Source: CAD feature listing. Evaluate the final solid. Frame: model axes, mm. Face numbers are marked on the shaded views. A direction names the side the tool comes from. Round coordinates to 2 decimals unless told otherwise and drop trailing zeros. Write each loop counter-clockwise with the first axis right and the second up, starting at its lowest first coordinate (ties: lowest second). Pieces come first, ordered by that corner, then holes. Notation, with made-up numbers: (1, 52) -> (11, 52) arc R16 cw to (11, 67) -> close; hole circle Ø7 at (31, 27.25). An arc over 180 degrees is marked (long way). Put each result on its own line as item: value.
```python
from build123d import *

# Parameters (mm, degrees)
BOSS_EXTRUDE1_DEPTH      = 3
BOSS_EXTRUDE2_START      = 22.115178
SKETCH3_W                = 10.4
SKETCH3_H                = 10.35
BOSS_EXTRUDE2_DEPTH      = 1
BOSS_EXTRUDE2_DEPTH_BACK = 3
CUT_EXTRUDE1_DEPTH       = 4
BOSS_EXTRUDE3_DEPTH      = 2
SKETCH6_W                = 4
SKETCH6_H                = 3.75
BOSS_EXTRUDE4_DEPTH      = 1
SKETCH7_W                = 4
SKETCH7_H                = 3.75
BOSS_EXTRUDE5_DEPTH      = 1
SKETCH8_W                = 3.8
SKETCH8_H                = 4
BOSS_EXTRUDE6_DEPTH      = 1
SKETCH9_W                = 3.8
SKETCH9_H                = 4
BOSS_EXTRUDE7_DEPTH      = 1
CUT_EXTRUDE2_DEPTH       = 3
BOSS_EXTRUDE8_DEPTH      = 3
BOSS_EXTRUDE9_DEPTH      = 6
BOSS_EXTRUDE10_DEPTH     = 7
SKETCH15_W               = 12.4
SKETCH15_H               = 12.35
CUT_EXTRUDE3_DEPTH       = 1.5


with BuildPart() as part:
    # Sketch1 → Boss-Extrude1 (new body)
    with BuildSketch(Plane.XY):
        Polygon((6.141518054, 8.123354813), (2.841518054, 8.123354813), (2.841518054, 5.623354813), (3.641518054, 4.823354813), (5.341518054, 4.823354813), (6.141518054, 5.623354813), align=None)
    extrude(amount=BOSS_EXTRUDE1_DEPTH)

    # Sketch3 → Boss-Extrude2 (add, two sides)
    with BuildSketch(Plane.XY.offset(-22.115178163).offset(BOSS_EXTRUDE2_START)) as boss_extrude2_sk:
        with Locations((4.491518054, 6.473354813)):
            Rectangle(SKETCH3_W, SKETCH3_H)
        Polygon((2.841518054, 8.123354813), (2.841518054, 5.623354813), (3.641518054, 4.823354813), (5.341518054, 4.823354813), (6.141518054, 5.623354813), (6.141518054, 8.123354813), align=None, mode=Mode.SUBTRACT)
    extrude(amount=BOSS_EXTRUDE2_DEPTH)
    extrude(boss_extrude2_sk.sketch, amount=-BOSS_EXTRUDE2_DEPTH_BACK)

    # Sketch4 → Cut-Extrude1 (cut)
    with BuildSketch(Plane.XY.offset(1)):
        with BuildLine():
            Line((-0.708481946, 4.598354813), (-0.708481946, 1.298354813))
            Line((-0.708481946, 1.298354813), (2.591518054, 1.298354813))
            ThreePointArc((2.591518054, 1.298354813), (1.624970432, 3.631807191), (-0.708481946, 4.598354813))
        make_face()
        with BuildLine():
            Line((9.691518054, 1.298354813), (6.391518054, 1.298354813))
            ThreePointArc((6.391518054, 1.298354813), (7.358065676, 3.631807191), (9.691518054, 4.598354813))
            Line((9.691518054, 4.598354813), (9.691518054, 1.298354813))
        make_face()
        with BuildLine():
            Line((9.691518054, 8.348354813), (9.691518054, 11.648354813))
            Line((9.691518054, 11.648354813), (6.391518054, 11.648354813))
            ThreePointArc((6.391518054, 11.648354813), (7.358065676, 9.314902435), (9.691518054, 8.348354813))
        make_face()
        with BuildLine():
            Line((-0.708481946, 8.348354813), (-0.708481946, 11.648354813))
            Line((-0.708481946, 11.648354813), (2.591518054, 11.648354813))
            ThreePointArc((2.591518054, 11.648354813), (1.624970432, 9.314902435), (-0.708481946, 8.348354813))
        make_face()
    extrude(amount=-CUT_EXTRUDE1_DEPTH, mode=Mode.SUBTRACT)

    # Sketch5 → Boss-Extrude3 (add)
    with BuildSketch(Plane.XY.offset(3)):
        Polygon((2.841518054, 5.623354813), (3.641518054, 4.823354813), (2.841518054, 4.823354813), align=None)
        Polygon((5.341518054, 4.823354813), (6.141518054, 5.623354813), (6.141518054, 4.823354813), align=None)
    extrude(amount=-BOSS_EXTRUDE3_DEPTH)

    # Sketch6 → Boss-Extrude4 (add)
    with BuildSketch(Plane.ZY.offset(0.708481946)):
        with Locations((-1, 6.473354813)):
            Rectangle(SKETCH6_W, SKETCH6_H)
    extrude(amount=BOSS_EXTRUDE4_DEPTH)

    # Sketch7 → Boss-Extrude5 (add)
    with BuildSketch(Plane(origin=(9.691518054, 0, 0), x_dir=(0, 0, -1), z_dir=(1, 0, 0))):
        with Locations((1, 6.473354813)):
            Rectangle(SKETCH7_W, SKETCH7_H)
    extrude(amount=BOSS_EXTRUDE5_DEPTH)

    # Sketch8 → Boss-Extrude6 (add)
    with BuildSketch(Plane(origin=(0, 11.648354813, 0), x_dir=(1, 0, 0), z_dir=(0, 1, 0))):
        with Locations((4.491518054, 1)):
            Rectangle(SKETCH8_W, SKETCH8_H)
    extrude(amount=BOSS_EXTRUDE6_DEPTH)

    # Sketch9 → Boss-Extrude7 (add)
    with BuildSketch(Plane.XZ.offset(-1.298354813)):
        with Locations((4.491518054, -1)):
            Rectangle(SKETCH9_W, SKETCH9_H)
    extrude(amount=BOSS_EXTRUDE7_DEPTH)

    # Sketch10 → Cut-Extrude2 (cut)
    with BuildSketch(Plane(origin=(0, 0, -3), x_dir=(-1, 0, 0), z_dir=(0, 0, -1))):
        Polygon((-6.641518054, 6.873354813), (-6.641518054, 8.623354813), (-4.491518054, 8.623354813), (-2.341518054, 8.623354813), (-2.341518054, 6.873354813), (-2.341518054, 5.623354813), (-3.641518054, 4.323354813), (-4.491518054, 4.323354813), (-5.341518054, 4.323354813), (-5.841518054, 4.823354813), (-6.641518054, 5.623354813), align=None)
    extrude(amount=-CUT_EXTRUDE2_DEPTH, mode=Mode.SUBTRACT)

    # Sketch11 → Boss-Extrude8 (add)
    with BuildSketch(Plane(origin=(0, 0, -3), x_dir=(-1, 0, 0), z_dir=(0, 0, -1))):
        with BuildLine():
            Line((0.708481946, 4.598354813), (1.708481946, 4.598354813))
            Line((1.708481946, 4.598354813), (1.708481946, 8.348354813))
            Line((1.708481946, 8.348354813), (0.708481946, 8.348354813))
            ThreePointArc((0.708481946, 8.348354813), (-1.624970432, 9.314902435), (-2.591518054, 11.648354813))
            Line((-2.591518054, 11.648354813), (-2.591518054, 12.648354813))
            Line((-2.591518054, 12.648354813), (-6.391518054, 12.648354813))
            Line((-6.391518054, 12.648354813), (-6.391518054, 11.648354813))
            ThreePointArc((-6.391518054, 11.648354813), (-7.358065676, 9.314902435), (-9.691518054, 8.348354813))
            Line((-9.691518054, 8.348354813), (-10.691518054, 8.348354813))
            Line((-10.691518054, 8.348354813), (-10.691518054, 4.598354813))
            Line((-10.691518054, 4.598354813), (-9.691518054, 4.598354813))
            ThreePointArc((-9.691518054, 4.598354813), (-7.358065676, 3.631807191), (-6.391518054, 1.298354813))
            Line((-6.391518054, 1.298354813), (-6.391518054, 0.298354813))
            Line((-6.391518054, 0.298354813), (-2.591518054, 0.298354813))
            Line((-2.591518054, 0.298354813), (-2.591518054, 1.298354813))
            ThreePointArc((-2.591518054, 1.298354813), (-1.624970432, 3.631807191), (0.708481946, 4.598354813))
        make_face()
        Polygon((-6.641518054, 5.623354813), (-5.341518054, 4.323354813), (-3.641518054, 4.323354813), (-2.341518054, 5.623354813), (-2.341518054, 8.623354813), (-6.641518054, 8.623354813), align=None, mode=Mode.SUBTRACT)
    extrude(amount=BOSS_EXTRUDE8_DEPTH)

    # Sketch13 → Boss-Extrude9 (add)
    with BuildSketch(Plane(origin=(0, 0, -6), x_dir=(-1, 0, 0), z_dir=(0, 0, -1))):
        Polygon((-2.341518054, 8.623354813), (-6.641518054, 8.623354813), (-6.641518054, 5.623354813), (-5.341518054, 4.323354813), (-3.641518054, 4.323354813), (-2.341518054, 5.623354813), align=None)
        Polygon((-6.391518054, 7.123354813), (-6.391518054, 8.373354813), (-4.491518054, 8.373354813), (-2.591518054, 8.373354813), (-2.591518054, 7.123354813), (-2.591518054, 5.726908204), (-3.168294749, 5.150131508), (-3.745071444, 4.573354813), (-4.491518054, 4.573354813), (-5.237964663, 4.573354813), (-5.814741358, 5.150131508), (-6.391518054, 5.726908204), align=None, mode=Mode.SUBTRACT)
    extrude(amount=-BOSS_EXTRUDE9_DEPTH)

    # Sketch14 → Boss-Extrude10 (add)
    with BuildSketch(Plane(origin=(0, 0, -6), x_dir=(-1, 0, 0), z_dir=(0, 0, -1))):
        Polygon((1.708481946, 4.598354813), (1.708481946, 8.348354813), (1.708481946, 12.648354813), (-2.591518054, 12.648354813), (-6.391518054, 12.648354813), (-10.691518054, 12.648354813), (-10.691518054, 8.348354813), (-10.691518054, 4.598354813), (-10.691518054, 0.298354813), (-6.391518054, 0.298354813), (-2.591518054, 0.298354813), (1.708481946, 0.298354813), align=None)
        Polygon((-6.391518054, 5.726908204), (-5.237964663, 4.573354813), (-3.745071444, 4.573354813), (-2.591518054, 5.726908204), (-2.591518054, 8.373354813), (-6.391518054, 8.373354813), align=None, mode=Mode.SUBTRACT)
    extrude(amount=-BOSS_EXTRUDE10_DEPTH)

    # Sketch15 → Cut-Extrude3 (cut)
    with BuildSketch(Plane(origin=(0, 0, -6), x_dir=(-1, 0, 0), z_dir=(0, 0, -1))):
        with Locations((-4.491518054, 6.473354813)):
            Rectangle(SKETCH15_W, SKETCH15_H)
    extrude(amount=-CUT_EXTRUDE3_DEPTH, mode=Mode.SUBTRACT)


solid = part.part
```
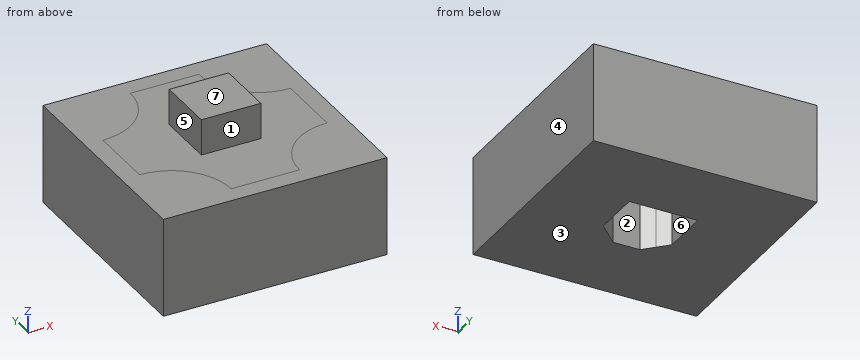
Q1. Pin query (flat end, axial travel): pin 1 (1.6 mm diameter, centred on y = 6, z = 1.5, fed in from +X); pin 2 (1.6 mm diameter, centred on y = 6.5, z = 2, fed in from -X); pin 3 (1.6 mm diameter, centred on x = 5, z = 2.5, fed in from -Y). Return the tip coordinate at first contact, or that it passes through.
Ans:
pin 1: stops at x = 10.69
pin 2: stops at x = 2.84
pin 3: stops at y = 4.82
Q2. Cut plane D-D on z = 1.75. Output: boundary loops of the cut face in (x, y).
Ans:
outline: (2.84, 4.82) -> (6.14, 4.82) -> (6.14, 8.12) -> (2.84, 8.12) -> close
Q3. Cut plane B-B on y = 6.25. Output: boundary loops of the cut face in (x, z).
Ans:
outline: (-1.71, -4.5) -> (2.59, -4.5) -> (2.59, 0) -> (6.39, 0) -> (6.39, -4.5) -> (10.69, -4.5) -> (10.69, 1) -> (6.14, 1) -> (6.14, 3) -> (2.84, 3) -> (2.84, 1) -> (-1.71, 1) -> close
Q4. Draft query along X for the marked faces 4, 5, 6 and 7. Return one class per face: +X half, -X half, draft (parallel to the pull), parting line (faces both ways), or undercut.
Ans:
face 4: +X half
face 5: -X half
face 6: undercut
face 7: draft
Q5. Cut plane C-C on x = 5. Output: boundary loops of the cut face in (y, z).
Ans:
outline: (0.3, -4.5) -> (4.57, -4.5) -> (4.57, 0) -> (8.37, 0) -> (8.37, -4.5) -> (12.65, -4.5) -> (12.65, 1) -> (8.12, 1) -> (8.12, 3) -> (4.82, 3) -> (4.82, 1) -> (0.3, 1) -> close
Q6. Reachability of the marked faces 1, 2 and 3 from +Z, -Z, +X, -X, +Y, -Y: full face, straight path, thin tool, end or side. Return the list, or none.
Ans:
face 1: +Z, +X, -X, -Y
face 2: -Z
face 3: -Z, +X, -X, +Y, -Y
Q7. Cut plane A-A on z = -3. Output: boundary loops of the cut face in (x, y).
Ans:
outline: (-1.71, 0.3) -> (10.69, 0.3) -> (10.69, 12.65) -> (-1.71, 12.65) -> close; hole (2.59, 5.73) -> (3.75, 4.57) -> (5.24, 4.57) -> (6.39, 5.73) -> (6.39, 8.37) -> (2.59, 8.37) -> close
Q8. Material intervals for line 1 (X direction, y = 5.75, z = -2); line 2 (Z direction, x = 5, y = 6.25); line 3 (Z direction, x = 5.75, y = 2.5), sorted ascending. Write a range as [from, to].
Ans:
line 1: x = [-1.71, 2.59], [6.39, 10.69]
line 2: z = [0, 3]
line 3: z = [-4.5, 1]
